Here's how the part is built. I have some questions about the finished solid (model axes, mm). A direction names the side the tool comes from. Round coordinates to 2 decimals unless told otherwise and drop trailing zeros. Loops run counter-clockwise (first coordinate to the right, second up) from the corner with the lowest first, then second, coordinate; pieces in that order, holes last. Notation, with made-up numbers: M 75.5,24 L 102.5,24 A18 cw 102.5,41 Z; hole C 40,-4 d3. An arc over 180 degrees is marked long. Write item = value, one per line. Start each with the question number.
from build123d import *

# Parameters (mm, degrees)
F0_R     = 25
F1_DEPTH = 15
F2_R     = 10
F3_DEPTH = 35
F4_R     = 3
F5_DEPTH = 15
F6_R     = 3
F7_DEPTH = 50
F8_R     = 5
F9_DEPTH = 10


with BuildPart() as f1:
    # F0 (on Top) → F1 (new body)
    with BuildSketch(Plane.XY):
        Circle(F0_R)
    extrude(amount=F1_DEPTH)

    # F2 (on face) → F3 (join)
    with BuildSketch(Plane.XY.offset(15)):
        Circle(F2_R)
    extrude(amount=F3_DEPTH)

    # F4 (on face) → F5 (cut)
    with BuildSketch(Plane.XY.offset(15)):
        with Locations((-17.5, 0)):
            Circle(F4_R)
        with Locations((17.5, 0)):
            Circle(F4_R)
    extrude(amount=-F5_DEPTH, mode=Mode.SUBTRACT)

    # F6 (on face) → F7 (cut)
    with BuildSketch(Plane.XY.offset(50)):
        Circle(F6_R)
    extrude(amount=-F7_DEPTH, mode=Mode.SUBTRACT)

    # F8 (on face) → F9 (cut)
    with BuildSketch(Plane.XY.offset(50)):
        Circle(F8_R)
    extrude(amount=-F9_DEPTH, mode=Mode.SUBTRACT)


solid = f1.part
Item 1: I want a section at B-B, the plane z = 17. List the corners of the cut face in (x, y) for me.
Item 2: We'd pull the mould along Y, two halves only. Please class faces 3 (the cylindrical face through (15.1, -1.8, 7.6)), 4 (the flat face through (0, -5, 0)), 5 (the cylindrical face through (-2.17, -9.76, 32.25)): released by +Y, released by -Y, zero draft, split by the parting line, or undercut.
Item 3: I want a section at A-A, the plane x = -17.5. List the corners of the cut face in (y, z) for me, then the cut area to 3 significant figures.
Item 4: I want a section at D-D, the plane x = 9. List the corners of the cut face in (y, z) for me, then the cut area to 3 significant figures.
Item 5: Will these pins go through, and if not, where does the flat tip stop? pin 1 Ø5 at (x, y) = (17.5, 0) entering from -Z; pin 2 Ø1.5 at (y, z) = (3.5, 12.5) entering from -X; pin 3 Ø2 at (y, z) = (18.5, 6) entering from +X; pin 4 Ø25 at (x, y) = (-10.5, 7) entering from +Z.
Item 6: For faces 1 (the cylindrical face through (23.846, 7.509, 7.395)), 2 (the flat face through (-0.1, -3.3, 40)), which set-ups out of +Z, -Z, +X, -X, +Y, -Y let a thin tool reach every point of the face, with its end or its side?
Item 7: I want a section at C-C, the plane y = -1. List the corners of the cut face in (x, z) for me.
Item 8: Please list where these lines run through material, in increasing order: line 1 (Y direction, x = 0, z = 47.5); line 2 (Z direction, x = -14, y = -1.5); line 3 (X direction, y = 1.5, z = 11). Write a range as [from, to].
Worked out:
q1.outline = C 0,0 d20; hole C 0,0 d6
q2.face_3 = undercut
q2.face_4 = zero draft
q2.face_5 = split by the parting line
q3.outline = M -17.85,0 L -3,0 L -3,15 L -17.85,15 Z; M 3,0 L 17.85,0 L 17.85,15 L 3,15 Z
q3.area = 446 mm2
q4.outline = M -23.32,0 L 23.32,0 L 23.32,15 L 4.36,15 L 4.36,50 L -4.36,50 L -4.36,15 L -23.32,15 Z
q4.area = 1,000 mm2
q5.pin_1 = through
q5.pin_2 = -24.85
q5.pin_3 = 17.85
q5.pin_4 = 50
q6.face_1 = +Z, -Z
q6.face_2 = +Z
q7.outline = M -24.98,0 L -20.33,0 L -20.33,15 L -24.98,15 Z; M -14.67,0 L -2.83,0 L -2.83,40 L -4.9,40 L -4.9,50 L -9.95,50 L -9.95,15 L -14.67,15 Z; M 2.83,0 L 14.67,0 L 14.67,15 L 9.95,15 L 9.95,50 L 4.9,50 L 4.9,40 L 2.83,40 Z; M 20.33,0 L 24.98,0 L 24.98,15 L 20.33,15 Z
q8.line_1 = [-10, -5], [5, 10]
q8.line_2 = [0, 15]
q8.line_3 = [-24.95, -20.1], [-14.9, -2.6], [2.6, 14.9], [20.1, 24.95]
